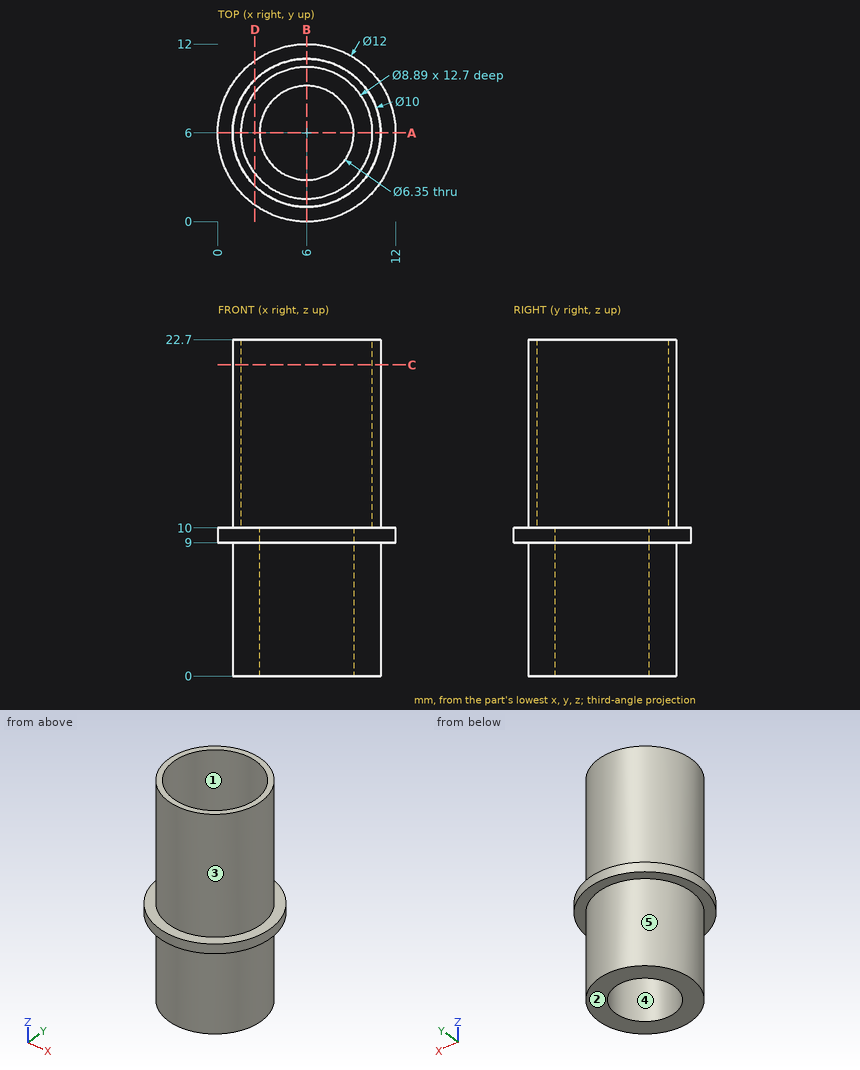
For this review, use the dimensioned drawing (mm, ordinates from the lowest corner) and the shaded views. A direction names the side the tool comes from. Coordinates: 2 decimals unless noted, no trailing zeros. Write each loop counter-clockwise with the first axis right and the second up, starting at its lowest first coordinate (ties: lowest second). Pieces come first, ordered by that corner, then holes. Notation, with made-up numbers: (89, -1.5) - (102, -1.5) arc R22 cw to (102, 26.5) - close; hole circle Ø6 at (74, 13). An arc over 180 degrees is marked (long way). One line per item, written item: value.
1) Add section D-D (x = 2.5). State the section outline as (y, z) points.
Answer sheet:
outline: (1.13, 9) - (2.43, 9) - (2.43, 0) - (9.57, 0) - (9.57, 9) - (10.87, 9) - (10.87, 10) - (9.57, 10) - (9.57, 22.7) - (8.74, 22.7) - (8.74, 10) - (3.26, 10) - (3.26, 22.7) - (2.43, 22.7) - (2.43, 10) - (1.13, 10) - close
2) To check wall thickness, follow probe 1 along Y at (x, z) = (6, 13) (3 decimals); probe 2 along Y at (x, z) = (6, 4.25) (3 decimals); probe 3 along X at (y, z) = (5, 13.75). State the ranges of each line that lie inside material, in increasing order.
Answer sheet:
probe 1: y = 1 to 1.555, 10.445 to 11
probe 2: y = 1 to 2.825, 9.175 to 11
probe 3: x = 1.1 to 1.67, 10.33 to 10.9
3) Mouldability with a two-part tool opening along Y and no side actions: class the marked faces 1, 2 and 3 as +Y half, -Y half, draft (parallel to the pull), parting line (faces both ways), or undercut.
Answer sheet:
face 1: undercut
face 2: draft
face 3: parting line
4) Insertion check: pin 1 (2 mm diameter, centred on y = 9.5, z = 14, fed in from -X); pin 2 (1 mm diameter, centred on y = 9.5, z = 19, fed in from +X); pin 3 (7 mm diameter, centred on x = 5.5, y = 6.5, fed in from +Z). Each pin has a flat end and moves straight along its axis. Give the tip position at first contact, or say it passes through.
Answer sheet:
pin 1: stops at x = 1.67
pin 2: stops at x = 10
pin 3: stops at z = 10
5) Add section A-A (y = 6). State the section outline as (x, z) points (3 decimals).
Answer sheet:
outline: (0, 9) - (1, 9) - (1, 0) - (2.825, 0) - (2.825, 10) - (1.555, 10) - (1.555, 22.7) - (1, 22.7) - (1, 10) - (0, 10) - close; (9.175, 0) - (11, 0) - (11, 9) - (12, 9) - (12, 10) - (11, 10) - (11, 22.7) - (10.445, 22.7) - (10.445, 10) - (9.175, 10) - close
6) Add section C-C (z = 21). State the section outline as (x, y) points (3 decimals).
Answer sheet:
outline: circle Ø10 at (6, 6); hole circle Ø8.89 at (6, 6)
7) For the marked faces 4 and 5, list the 3-axis set-ups (+Z, -Z, +X, -X, +Y, -Y) from which the entire face can be reached by the end or side of a thin tool; tool diameter is ignored.
Answer sheet:
face 4: +Z, -Z
face 5: -Z
